Here's how the part is built. I have some questions about the finished solid (model axes, mm). A direction names the side the tool comes from. Coordinates: 2 decimals unless noted, no trailing zeros. Order: outer loops, then holes, each group sorted by start corner. A loop starts at its lowest first (then second) coordinate and runs counter-clockwise, first axis right, second up. Notation, with made-up numbers: (63.5, 40.25) - (72.5, 40.25) arc R21 cw to (72.5, 56.25) - close; hole circle Ø11 at (25.5, 13.25). An arc over 180 degrees is marked (long way). Answer as CSV lines item,"result". Start each with the question number.
Q1. Suppose I cut it at B-B (z = 1.5). Please give me the cut outline in (x, y), then the cut area to 3 significant figures.
Q2. I need wall thicknesses on line 1 (X direction, y = 1.75, z = 0.5); line 2 (Z direction, x = 27.5, y = 2); line 3 (Y direction, x = -19, z = 6). Which ranges of each line are inside material? Lowest first, please.
Q3. For faces 1 (the face through (-33, 6, 0)), 2 (the face through (0, 10, 0)), which set-ups out of +Z, -Z, +X, -X, +Y, -Y let a thin tool reach every point of the face, with its end or its side?
Q4. Suppose I cut it at A-A (y = 6.25). Please give me the cut outline in (x, z), then the cut area to 3 significant figures.
Q5. Suppose I cut it at C-C (x = 24.5). Please give me the cut outline in (y, z).
Q6. Thinking about a two-plate mould opening in Z: for faces 3 (the face through (0, 6, -21)), 4 (the face through (-30, 5, 0)), 5 (the face through (-3, 0, 19)), 6 (the face through (0, 6, 21)), which applies, released by +Z, released by -Z, zero draft, split by the parting line, or undercut?
Q7. For pin 1 Ø18 at (x, z) = (5, 5.5) entering from -Y, with a flat end and sliding along its axis, tell me the tip position at first contact or that it passes through.
from build123d import *

# Parameters (mm, degrees)
SKETCH1_W           = 66
SKETCH1_H           = 42
SKETCH1_W_2         = 60
SKETCH1_H_2         = 36
BOSS_EXTRUDE1_DEPTH = 10
SKETCH3_W           = 66
SKETCH3_H           = 42
BOSS_EXTRUDE3_DEPTH = 3
FILLET2_R           = 1


with BuildPart() as part:
    # Sketch1 → Boss-Extrude1 (new body)
    with BuildSketch(Plane(origin=(0, 0, 0), x_dir=(1, 0, 0), z_dir=(0, 1, 0))):
        Rectangle(SKETCH1_W, SKETCH1_H)
        Rectangle(SKETCH1_W_2, SKETCH1_H_2, mode=Mode.SUBTRACT)
    extrude(amount=BOSS_EXTRUDE1_DEPTH)

    # Sketch3 → Boss-Extrude3 (add)
    with BuildSketch(Plane(origin=(0, 10, 0), x_dir=(1, 0, 0), z_dir=(0, 1, 0))):
        Rectangle(SKETCH3_W, SKETCH3_H)
    extrude(amount=BOSS_EXTRUDE3_DEPTH)

    # Fillet2
    fillet2_edges = [part.edges().sort_by_distance(p)[0] for p in [
        (-33, 13, 0),
        (0, 13, 21),
        (33, 13, 0),
        (0, 13, -21),
    ]]
    fillet(fillet2_edges, radius=FILLET2_R)


solid = part.part
Here are the results:
1,outline,"(-33, 0) - (-30, 0) - (-30, 10) - (30, 10) - (30, 0) - (33, 0) - (33, 12) arc R1 ccw to (32, 13) - (-32, 13) arc R1 ccw to (-33, 12) - close"
1,area,"258 mm²"
2,line 1,"x = -33 to -30, 30 to 33"
2,line 2,"z = -21 to -18, 18 to 21"
2,line 3,"y = 10 to 13"
3,face 1,"+Z, -Z, -X, +Y, -Y"
3,face 2,"-Y"
4,outline,"(-33, -21) - (33, -21) - (33, 21) - (-33, 21) - close; hole (-30, -18) - (30, -18) - (30, 18) - (-30, 18) - close"
4,area,"612 mm²"
5,outline,"(0, -21) - (12, -21) arc R1 ccw to (13, -20) - (13, 20) arc R1 ccw to (12, 21) - (0, 21) - (0, 18) - (10, 18) - (10, -18) - (0, -18) - close"
6,face 3,"released by -Z"
6,face 4,"undercut"
6,face 5,"zero draft"
6,face 6,"released by +Z"
7,pin 1,"stops at y = 10"
